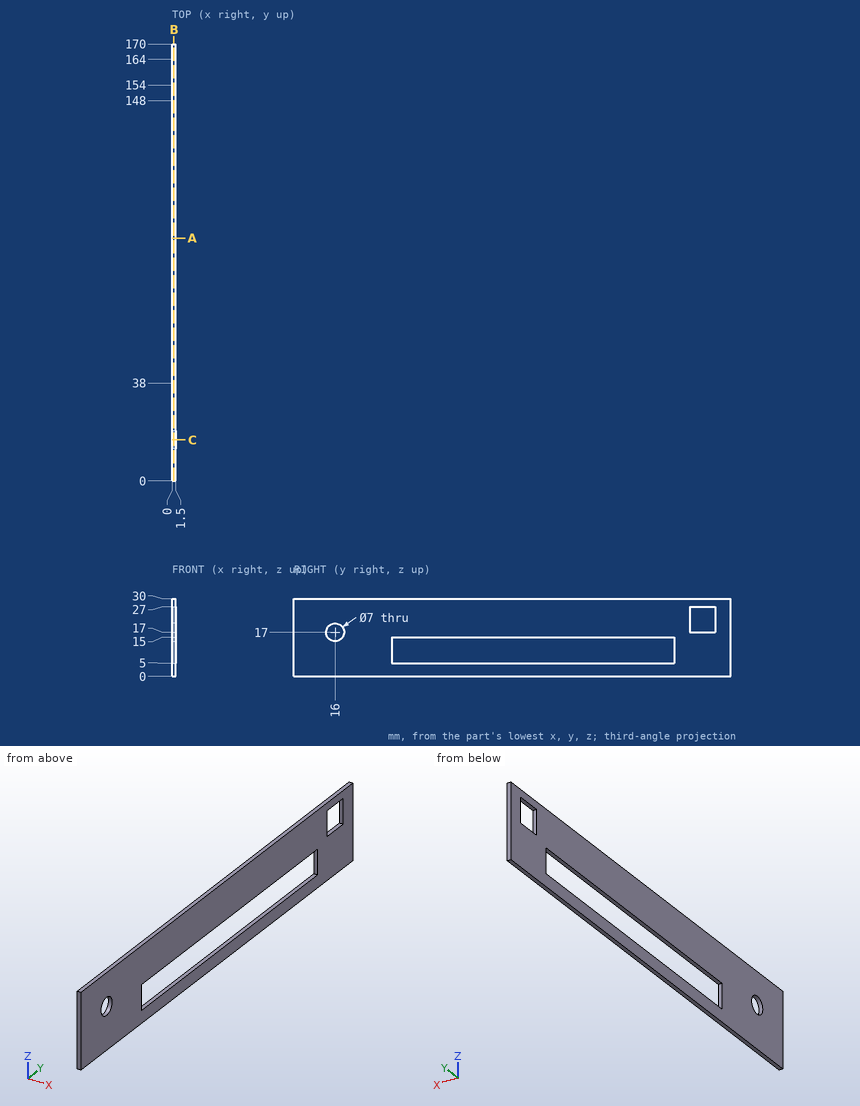
The figure shows three views and two pictorial views of one solid part (mm, origin at its lowest corner). Answer the questions. Coordinates: 2 decimals unless noted, no trailing zeros. Loops run counter-clockwise (first coordinate to the right, second up) from the corner with the lowest first, then second, coordinate; pieces in that order, holes last. Notation, with made-up numbers: (53.25, -20.5) -> (80.25, -20.5) arc R18 cw to (80.25, -11.5) -> close; hole circle Ø10 at (60.25, 40.5). An arc over 180 degrees is marked (long way). Return JSON: item names as keys, results as strings. Group by question number.
(1) A cutting plane is placed at B-B on x = 0.7. Write down the section's boundary in (y, z).
(2) Find the intervals of material crossed by probe 1 along Z at (x, y) = (0.9, 16); probe 2 along Z at (x, y) = (1.2, 147.5); probe 3 along Y at (x, z) = (1.15, 18), in increasing order. Write a range as from..to.
(3) A cutting plane is placed at C-C on y = 16. Write down the section's boundary in (x, z), and give its area (3 significant figures).
(4) A cutting plane is placed at A-A on y = 94.5. Write down the section's boundary in (x, z), and give its area (3 significant figures).
The answers:
{
 "1": {"outline": "(0, 0) -> (170, 0) -> (170, 30) -> (0, 30) -> close; hole circle Ø7 at (16, 17); hole (38, 5) -> (148, 5) -> (148, 15) -> (38, 15) -> close; hole (154, 17) -> (164, 17) -> (164, 27) -> (154, 27) -> close"},
 "2": {"probe 1": "z = 0..13.5, 20.5..30", "probe 2": "z = 0..5, 15..30", "probe 3": "y = 0..12.65, 19.35..154, 164..170"},
 "3": {"outline": "(0, 0) -> (1.5, 0) -> (1.5, 13.5) -> (0, 13.5) -> close; (0, 20.5) -> (1.5, 20.5) -> (1.5, 30) -> (0, 30) -> close", "area": "34.5 mm^2"},
 "4": {"outline": "(0, 0) -> (1.5, 0) -> (1.5, 5) -> (0, 5) -> close; (0, 15) -> (1.5, 15) -> (1.5, 30) -> (0, 30) -> close", "area": "30.0 mm^2"}
}
